Geometry: see drawing. Coordinates: mm, zero at the bounding-box minimum. A direction names the side the tool comes from. Give positions to 0.01 mm unless a question says otherwise; leave off trailing zeros. Loops run counter-clockwise (first coordinate to the right, second up) from the corner with the lowest first, then second, coordinate; pieces in that order, holes last. Notation, with made-up numbers: (-17, -0.5) - (24, -0.5) arc R8 ccw to (24, 7.5) - close; hole circle Ø9 at (48, 16). An arc over 180 degrees is marked (long way). Use one line per item in the form item = value.
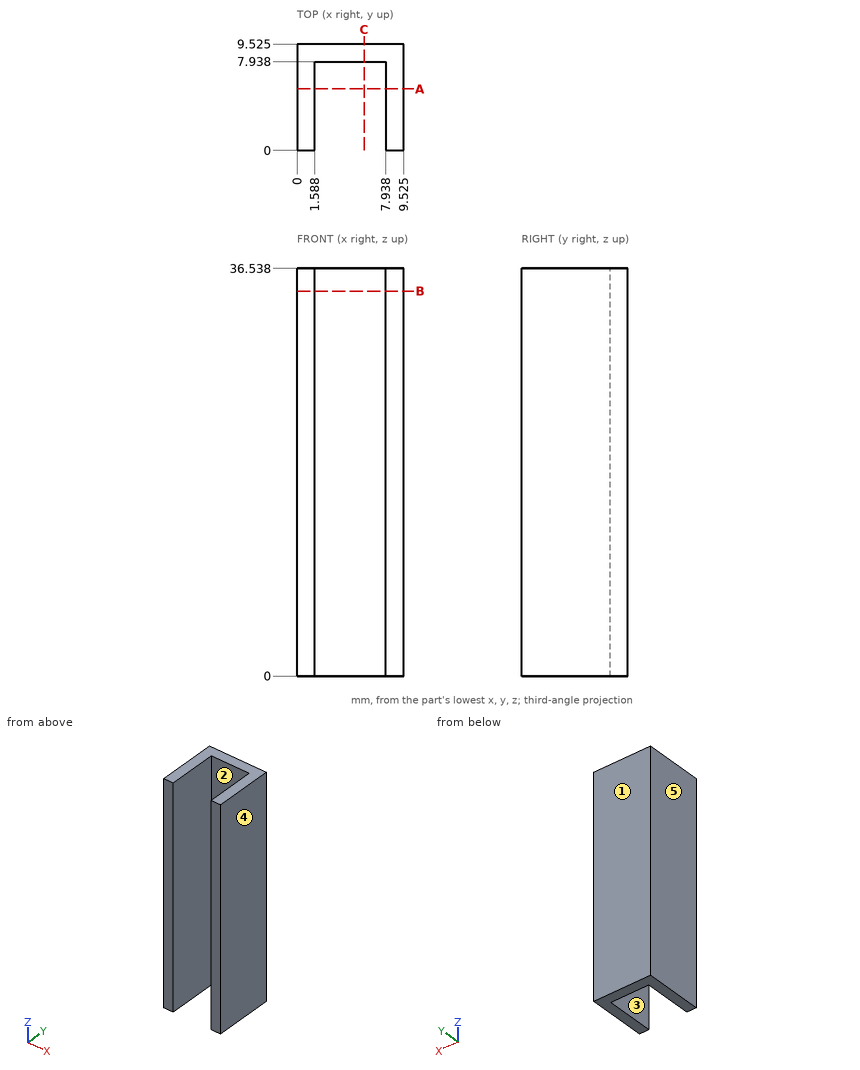
(1) Cut plane C-C (x = 6). Return the cut outline in (y, z) (1 decimal).
Solution:
outline = (7.9, 0) - (9.5, 0) - (9.5, 36.5) - (7.9, 36.5) - close
(2) Cut plane B-B (z = 34.5). Return the cut outline in (x, y) (1 decimal).
Solution:
outline = (0, 0) - (1.6, 0) - (1.6, 7.9) - (7.9, 7.9) - (7.9, 0) - (9.5, 0) - (9.5, 9.5) - (0, 9.5) - close
(3) Material intervals for L1, parallel to X at y = 6.5, z = 17 (1 decimal); L2, parallel to Y at x = 4.5, z = 26 (1 decimal), sorted ascending. Write a range as from..to.
Solution:
L1 = 0..1.6, 7.9..9.5
L2 = 7.9..9.5
(4) Cut plane A-A (y = 5.5). Return the cut outline in (x, z) (1 decimal).
Solution:
outline = (0, 0) - (1.6, 0) - (1.6, 36.5) - (0, 36.5) - close; (7.9, 0) - (9.5, 0) - (9.5, 36.5) - (7.9, 36.5) - close
(5) Pull-direction query (X, two-part tool) for the marked faces 3, 4 and 5; classes: released by +X, released by -X, zero draft, split by the parting line, or undercut.
Solution:
face_3 = undercut
face_4 = released by +X
face_5 = released by -X
(6) Access query for the marked faces 1 and 2. Directions: +Z, -Z, +X, -X, +Y, -Y. A direction counts if a zero-diameter tool reaches every point of the face in a straight line with its end or side. Return the directions, or none.
Solution:
face_1 = +Z, -Z, +X, -X, +Y
face_2 = +Z, -Z, -Y
